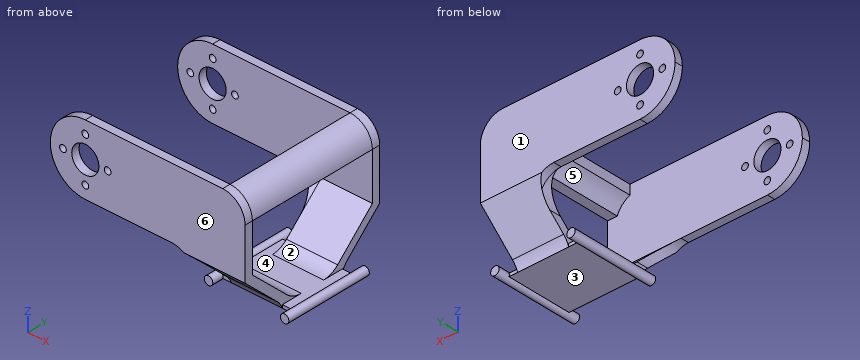
```python
from build123d import *

# Parameters (mm, degrees)
SKETCH1_W           = 23.83
SKETCH1_H           = 1
BOSS_EXTRUDE1_DEPTH = 20.5
SKETCH2_R           = 1.325
BOSS_EXTRUDE2_DEPTH = 13.75
BOSS_EXTRUDE4_DEPTH = 8
SKETCH5_W           = 21.919818374
SKETCH5_H           = 2.5
BOSS_EXTRUDE5_DEPTH = 45
SKETCH6_R           = 4.25
SKETCH6_R_2         = 1.05
CUT_EXTRUDE1_DEPTH  = 79.646360374
FILLET1_R           = 7
FILLET2_R           = 7
FILLET3_R           = 7
BOSS_EXTRUDE6_START = 41
BOSS_EXTRUDE6_DEPTH = 41


with BuildPart() as part:
    # Sketch1 → Boss-Extrude1 (new body)
    with BuildSketch(Plane(origin=(0, 0, 0), x_dir=(1, 0, 0), z_dir=(0, 1, 0))):
        Rectangle(SKETCH1_W, SKETCH1_H)
    extrude(amount=BOSS_EXTRUDE1_DEPTH)

    # Sketch2 → Boss-Extrude2 (add, symmetric)
    with BuildSketch(Plane(origin=(0, 10.25, 0), x_dir=(1, 0, 0), z_dir=(0, 1, 0))):
        with Locations(Location((-11.915, 0, 0), (0, 0, 270))):
            Circle(SKETCH2_R)
        with Locations(Location((11.915, 0, 0), (0, 0, 270))):
            Circle(SKETCH2_R)
    extrude(amount=BOSS_EXTRUDE2_DEPTH, both=True)

    # Sketch4 → Boss-Extrude4 (add, symmetric)
    with BuildSketch(Plane(origin=(0, 0, 0), x_dir=(0, 0, -1), z_dir=(1, 0, 0))):
        Polygon((-0.5, 16.852307022), (-0.5, 20.5), (-12.5, 33.25), (-35.5, 33.25), (-35.5, 30.75), (-13.580181626, 30.75), align=None)
        Polygon((-0.5, 0), (-0.5, 3.647692978), (-13.580181626, -10.25), (-35.5, -10.25), (-35.5, -12.75), (-12.5, -12.75), align=None)
    extrude(amount=BOSS_EXTRUDE4_DEPTH, both=True)

    # Sketch5 → Boss-Extrude5 (add)
    with BuildSketch(Plane.ZY.offset(8)):
        with Locations((24.540090813, 32)):
            Rectangle(SKETCH5_W, SKETCH5_H)
        with Locations((24.540090813, -11.5)):
            Rectangle(SKETCH5_W, SKETCH5_H)
    extrude(amount=BOSS_EXTRUDE5_DEPTH)

    # Sketch6 → Cut-Extrude1 (cut, through all)
    with BuildSketch(Plane(origin=(0, 33.25, 0), x_dir=(1, 0, 0), z_dir=(0, 1, 0))):
        with Locations(Location((-42.040090813, -24.540090813, 0), (0, 0, 270))):
            Circle(SKETCH6_R)
        with Locations(Location((-49.040090813, -24.540090813, 0), (0, 0, 270))):
            Circle(SKETCH6_R_2)
        with Locations(Location((-42.040090813, -17.540090813, 0), (0, 0, 270))):
            Circle(SKETCH6_R_2)
        with Locations(Location((-35.040090813, -24.540090813, 0), (0, 0, 270))):
            Circle(SKETCH6_R_2)
        with Locations(Location((-42.040090813, -31.540090813, 0), (0, 0, 270))):
            Circle(SKETCH6_R_2)
        with BuildLine():
            ThreePointArc((-53, -24.540090813), (-49.78991692, -16.790264706), (-42.040090813, -13.580181626))
            Line((-42.040090813, -13.580181626), (-53, -13.580181626))
            Line((-53, -13.580181626), (-53, -24.540090813))
        make_face()
        with BuildLine():
            ThreePointArc((-42.040090813, -35.5), (-49.78991692, -32.28991692), (-53, -24.540090813))
            Line((-53, -24.540090813), (-53, -35.5))
            Line((-53, -35.5), (-42.040090813, -35.5))
        make_face()
    extrude(amount=-CUT_EXTRUDE1_DEPTH, mode=Mode.SUBTRACT)

    # Fillet1
    # the kernel refuses this fillet: 7 mm, written as the material it adds along each edge
    with BuildSketch(Plane(origin=(-8, -12.75, 13.580181626), x_dir=(-1, 0, 0), z_dir=(0, 1, 0))) as fillet1_piece_1_section:
        with BuildLine():
            CenterArc((FILLET1_R, -FILLET1_R), FILLET1_R, 90, 90)
            Line((0, -FILLET1_R), (0, 0))
            Line((0, 0), (FILLET1_R, 0))
        make_face()
    fillet1_piece_1 = extrude(amount=2.5, mode=Mode.PRIVATE)
    fillet1_piece_1 = split(fillet1_piece_1, bisect_by=Plane(origin=(-10.020174451, -12.153760937, 11.938833823), z_dir=(0, 0.6853646990049913, 0.7281999926928027)), keep=Keep.TOP, mode=Mode.PRIVATE)
    fillet1_piece_1 = split(fillet1_piece_1, bisect_by=Plane(origin=(-10.020174451, -10.440349189, 13.759333804), z_dir=(0, -0.685364699004991, -0.7281999926928029)), keep=Keep.TOP, mode=Mode.PRIVATE)
    add(fillet1_piece_1)
    with BuildSketch(Plane(origin=(-8, -12.75, 13.580181626), x_dir=(-1, 0, 0), z_dir=(0, 1, 0))) as fillet1_piece_2_section:
        with BuildLine():
            CenterArc((FILLET1_R, -FILLET1_R), FILLET1_R, 90, 90)
            Line((0, -FILLET1_R), (0, 0))
            Line((0, 0), (FILLET1_R, 0))
        make_face()
    fillet1_piece_2 = extrude(amount=20, mode=Mode.PRIVATE)
    fillet1_piece_2 = split(fillet1_piece_2, bisect_by=Plane(origin=(-8.816209607, -9.698679662, 9.628169093), z_dir=(0, 0.6853646990049913, 0.7281999926928027)), keep=Keep.TOP, mode=Mode.PRIVATE)
    fillet1_piece_2 = split(fillet1_piece_2, bisect_by=Plane(origin=(-8.816209607, -10.25, 10.809130305), z_dir=(0, 1, 0)), keep=Keep.TOP, mode=Mode.PRIVATE)
    fillet1_piece_2 = split(fillet1_piece_2, bisect_by=Plane(origin=(-8.816209607, -7.985267914, 11.448669075), z_dir=(0, -0.685364699004991, -0.7281999926928029)), keep=Keep.TOP, mode=Mode.PRIVATE)
    add(fillet1_piece_2)
    with BuildSketch(Plane(origin=(-8, 33.25, 13.580181626), x_dir=(0, 0, -1), z_dir=(0, -1, 0))) as fillet1_piece_3_section:
        with BuildLine():
            CenterArc((FILLET1_R, -FILLET1_R), FILLET1_R, 90, 90)
            Line((0, -FILLET1_R), (0, 0))
            Line((0, 0), (FILLET1_R, 0))
        make_face()
    fillet1_piece_3 = extrude(amount=2.5, mode=Mode.PRIVATE)
    fillet1_piece_3 = split(fillet1_piece_3, bisect_by=Plane(origin=(-10.020174451, 32.653760936, 11.938833823), z_dir=(0, -0.6853646990049912, 0.7281999926928028)), keep=Keep.TOP, mode=Mode.PRIVATE)
    fillet1_piece_3 = split(fillet1_piece_3, bisect_by=Plane(origin=(-10.020174451, 30.940349189, 13.759333804), z_dir=(0, 0.6853646990049909, -0.7281999926928031)), keep=Keep.TOP, mode=Mode.PRIVATE)
    add(fillet1_piece_3)
    with BuildSketch(Plane(origin=(-8, 33.25, 13.580181626), x_dir=(0, 0, -1), z_dir=(0, -1, 0))) as fillet1_piece_4_section:
        with BuildLine():
            CenterArc((FILLET1_R, -FILLET1_R), FILLET1_R, 90, 90)
            Line((0, -FILLET1_R), (0, 0))
            Line((0, 0), (FILLET1_R, 0))
        make_face()
    fillet1_piece_4 = extrude(amount=20, mode=Mode.PRIVATE)
    fillet1_piece_4 = split(fillet1_piece_4, bisect_by=Plane(origin=(-8.816209616, 30.198679665, 9.628169097), z_dir=(0, -0.6853646990049912, 0.7281999926928028)), keep=Keep.TOP, mode=Mode.PRIVATE)
    fillet1_piece_4 = split(fillet1_piece_4, bisect_by=Plane(origin=(-8.816209616, 28.485267918, 11.448669078), z_dir=(0, 0.6853646990049909, -0.7281999926928031)), keep=Keep.TOP, mode=Mode.PRIVATE)
    fillet1_piece_4 = split(fillet1_piece_4, bisect_by=Plane(origin=(-8.816209616, 30.75, 10.809130308), z_dir=(0, -1, 0)), keep=Keep.TOP, mode=Mode.PRIVATE)
    add(fillet1_piece_4)
    # the kernel refuses this fillet: 7 mm, written as the material it takes off along each edge
    with BuildSketch(Plane(origin=(8, 7.25, 35.5), x_dir=(0, 0, -1), z_dir=(0, -1, 0))) as fillet1_2_piece_1:
        with BuildLine():
            CenterArc((FILLET1_R, -FILLET1_R), FILLET1_R, 90, 90)
            Line((0, -FILLET1_R), (0, 0))
            Line((0, 0), (FILLET1_R, 0))
        make_face()
    extrude(amount=37.5, mode=Mode.SUBTRACT)
    with BuildSketch(Plane(origin=(8, 50.75, 35.5), x_dir=(-1, 0, 0), z_dir=(0, -1, 0))) as fillet1_2_piece_2:
        with BuildLine():
            CenterArc((FILLET1_R, FILLET1_R), FILLET1_R, 180, 90)
            Line((0, FILLET1_R), (0, 0))
            Line((0, 0), (FILLET1_R, 0))
        make_face()
    extrude(amount=37.5, mode=Mode.SUBTRACT)

    # Fillet2
    fillet2_edges = [part.edges().sort_by_distance(p)[0] for p in [
        (0, 16.852307022, 0.5),
        (0, 3.647692978, 0.5),
    ]]
    fillet(fillet2_edges, radius=FILLET2_R)

    # Fillet3
    # the kernel refuses this fillet: 7 mm, written as the material it adds along each edge
    with BuildSketch(Plane(origin=(-8, 20.5, 0.5), x_dir=(0, 0.7281999926925888, 0.6853646990052185), z_dir=(1, 0, 0))) as fillet3_piece_1:
        with BuildLine():
            CenterArc((2.423417163, -7), FILLET3_R, 90, 26.366519243)
            Line((-0.685364699, -0.728199993), (0, 0))
            Line((0, 0), (2.423417163, 0))
        make_face()
    extrude(amount=16)
    with BuildSketch(Plane(origin=(8, 0, 0.5), x_dir=(0, 0, -1), z_dir=(-1, 0, 0))) as fillet3_piece_2:
        with BuildLine():
            CenterArc((3.436475374, 6.562285254), FILLET3_R, 223.264295411, 26.366519243)
            Line((-1.660924575, 1.764732361), (0, 0))
            Line((0, 0), (1, 0))
        make_face()
    extrude(amount=16)

    # Sketch8 → Boss-Extrude6 (add)
    with BuildSketch(Plane(origin=(0, -10.25, 0), x_dir=(1, 0, 0), z_dir=(0, 1, 0)).offset(BOSS_EXTRUDE6_START)):
        with BuildLine():
            ThreePointArc((1, -35.5), (5.949747468, -33.449747468), (8, -28.5))
            Line((8, -28.5), (5, -28.5))
            ThreePointArc((5, -28.5), (3.422054899, -30.922054899), (1, -32.5))
            Line((1, -32.5), (1, -35.5))
        make_face()
    extrude(amount=-BOSS_EXTRUDE6_DEPTH)


solid = part.part
```
Work out the finished part from the listing and answer in its coordinate system (mm). Face numbers are marked on the shaded views. A direction names the side the tool comes from. Coordinates: 2 decimals unless noted, no trailing zeros. Loops run counter-clockwise (first coordinate to the right, second up) from the corner with the lowest first, then second, coordinate; pieces in that order, holes last. Notation, with made-up numbers: M 75.25,1 L 117.25,1 A28 cw 117.25,25 Z; hole C -16.5,65.25 d9. An arc over 180 degrees is marked long. Use CSV: the item, a comma, the result in double quotes. Start each with the question number.
(1) Find section B-B, the plane x = -22. Give the vertices of the cut face in (y, z), then the cut area to 3 significant figures.
(2) Consider line 1 (Y direction, x = -33.5, z = 27.5); line 2 (Z direction, x = 5.5, y = 23); line 3 (Y direction, x = 3, z = 12). Determine where each line is inside the solid, lowest interval first.
(3) Find section C-C, the plane x = 7. Give the vertices of the cut face in (y, z), then the cut area to 3 significant figures.
(4) For a pull along Z with two mould halves and no side action, classify the marked faces 1, 2 and 3 as +Z half, -Z half, draft (parallel to the pull), parting line (faces both ways), or undercut.
(5) Given pin 1 Ø0.8 at (x, z) = (10, 0) entering from -Y; pin 2 Ø3.5 at (y, z) = (19.5, 4.5) entering from -X; pin 3 Ø0.8 at (x, z) = (-12, 0) entering from +Y, each flat-ended and moving along its own axis, determine where each tip first touches the part or whether it passes through.
(6) Find section A-A, the plane y = 8. Give the vertices of the cut face in (x, z) (3 decimals).
(7) For the marked faces 4, 5 and 6, determine the directions among +Z, -Z, +X, -X, +Y, -Y from which every point of the face is accessible in a straight line to the end or side of a thin tool.
(8) Find section D-D, the plane y = 17. Give the vertices of the cut face in (x, z) (3 decimals).
Recorded:
1,outline,"M -12.75,13.58 L -10.25,13.58 L -10.25,35.5 L -12.75,35.5 Z; M 30.75,13.58 L 33.25,13.58 L 33.25,35.5 L 30.75,35.5 Z"
1,area,"110 mm^2"
2,line 1,"y = -12.75 to -10.25, 30.75 to 33.25"
2,line 2,"z = 2.85 to 6.29, 28.5 to 33.86"
2,line 3,"y = -12.22 to -8.57, 29.07 to 32.72"
3,outline,"M -12.75,12.5 L -1.76,2.16 A7 cw 0,-0.5 L 20.5,-0.5 A7 cw 22.26,2.16 L 33.25,12.5 L 33.25,32.11 L -12.75,32.11 Z; hole M -10.25,13.58 L 1.63,2.4 A7 ccw 6.42,0.5 L 14.08,0.5 A7 ccw 18.87,2.4 L 30.75,13.58 L 30.75,28.5 L -10.25,28.5 Z"
3,area,"358 mm^2"
4,face 1,"draft"
4,face 2,"undercut"
4,face 3,"-Z half"
5,pin 1,"stops at y = 0"
5,pin 2,"stops at x = -8"
5,pin 3,"stops at y = 24"
6,outline,"M -10.688,-0.5 L 10.688,-0.5 A1.325 ccw long 10.688,0.5 L -10.688,0.5 A1.325 ccw long Z; M 1,32.5 A7 cw 5,28.5 L 8,28.5 A7 ccw 1,35.5 Z"
7,face 4,"none"
7,face 5,"-X"
7,face 6,"+Z, -Z, +X, -X, -Y"
8,outline,"M -10.688,-0.5 L 10.688,-0.5 A1.325 ccw long 10.688,0.5 L 8,0.5 L 8,1.14 L -8,1.14 L -8,0.5 L -10.688,0.5 A1.325 ccw long Z; M 1,32.5 A7 cw 5,28.5 L 8,28.5 A7 ccw 1,35.5 Z"
